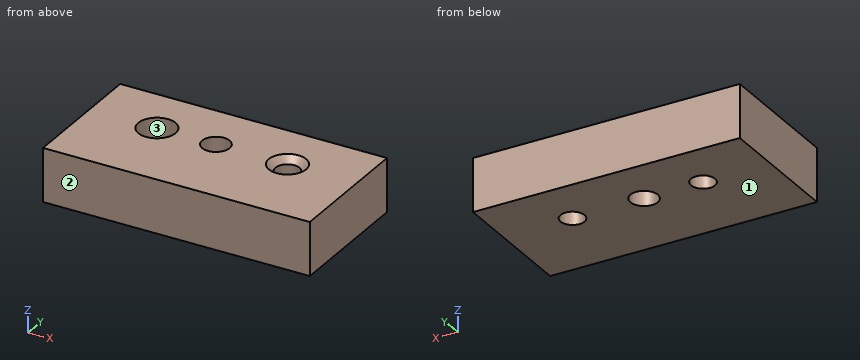
```python
from build123d import *

# Parameters (mm, degrees)
F0_W           = 100
F0_H           = 50
F1_DEPTH       = 20
F3_D           = 9
F3_DEPTH       = 30
F3_CBORE_D     = 14
F3_CBORE_DEPTH = 10
F3_TIP         = 2.7038727856
F4_D           = 9
F4_CSINK_D     = 14
F4_CSINK_ANGLE = 90
F5_D           = 10.3


with BuildPart() as f1:
    # F0 (on Top) → F1 (new body)
    with BuildSketch(Plane.XY):
        with Locations((19.3940885365, -5.1782257724)):
            Rectangle(F0_W, F0_H)
    extrude(amount=F1_DEPTH)

    # F3
    with Locations(Plane.XY.offset(20)):
        with Locations((-5.3611323237, 0)):
            CounterBoreHole(F3_D / 2, F3_CBORE_D / 2, F3_CBORE_DEPTH, depth=F3_DEPTH)
            with Locations((0, 0, -(F3_DEPTH + F3_TIP / 2))):  # 118° drill point
                Cone(0, F3_D / 2, F3_TIP, mode=Mode.SUBTRACT)

    # F4 (through all)
    with Locations(Plane.XY.offset(20)):
        with Locations((43.5566157103, 0)):
            CounterSinkHole(F4_D / 2, F4_CSINK_D / 2, counter_sink_angle=F4_CSINK_ANGLE)

    # F5 (through all)
    with Locations(Plane.XY.offset(20)):
        with Locations((16.7399458587, 0)):
            Hole(F5_D / 2)


solid = f1.part
```
Model file for the job. Use its own axes, mm. Face numbers are marked on the shaded views. Coordinates: 2 decimals unless noted, no trailing zeros. Order: outer loops, then holes, each group sorted by start corner. A loop starts at its lowest first (then second) coordinate and runs counter-clockwise, first axis right, second up. Notation, with made-up numbers: (55.5, 6.5) - (87.5, 6.5) arc R30 cw to (87.5, 34.5) - close; hole circle Ø7 at (55.25, -5). An arc over 180 degrees is marked (long way). Return JSON: item names as keys, results as strings. Group by question number.
1) Saw through at B-B, the plane z = 6.5. Write the cut outline in (x, y).
2) Saw through at A-A, the plane y = 0. Write the cut outline in (x, z), plus the area to 3 significant figures.
3) Saw through at C-C, the plane z = 15.25. Write the cut outline in (x, y), plus the area to 3 significant figures.
4) Flat gauge pins, fed straight in: P1, Ø8, axis at x = -5.36, y = 0, coming from the +Z side; P2, Ø7, axis at x = -6, y = 2, coming from the +Z side. Where does each tip first touch, or does it go through?
5) Mould opens along Y. For the marked faces 1, 2 and 3 say: released by +Y, released by -Y, zero draft, split by the parting line, or undercut.
6) Probe line 1 (X direction, y = -4, z = 17); line 2 (Y direction, x = 43, z = 5.25); line 3 (Y direction, x = 13.5, z = 14.5). List the from-to ranges inside material, lowest first. Write a range as from..to.
7) Saw through at D-D, the plane x = 0.5. Write the cut outline in (y, z).
Values found:
{
 "1": {"outline": "(-30.61, -30.18) - (69.39, -30.18) - (69.39, 19.82) - (-30.61, 19.82) - close; hole circle Ø9 at (-5.36, 0); hole circle Ø10.3 at (16.74, 0); hole circle Ø9 at (43.56, 0)"},
 "2": {"outline": "(-30.61, 0) - (-9.86, 0) - (-9.86, 10) - (-12.36, 10) - (-12.36, 20) - (-30.61, 20) - close; (-0.86, 0) - (11.59, 0) - (11.59, 20) - (1.64, 20) - (1.64, 10) - (-0.86, 10) - close; (21.89, 0) - (39.06, 0) - (39.06, 17.5) - (36.56, 20) - (21.89, 20) - close; (48.06, 0) - (69.39, 0) - (69.39, 20) - (50.56, 20) - (48.06, 17.5) - close", "area": "1,380 mm²"},
 "3": {"outline": "(-30.61, -30.18) - (69.39, -30.18) - (69.39, 19.82) - (-30.61, 19.82) - close; hole circle Ø14 at (-5.36, 0); hole circle Ø10.3 at (16.74, 0); hole circle Ø9 at (43.56, 0)", "area": "4,700 mm²"},
 "4": {"P1": "passes through", "P2": "stops at z = 10"},
 "5": {"face 1": "zero draft", "face 2": "released by -Y", "face 3": "undercut"},
 "6": {"line 1": "x = -30.61..-11.11, 0.38..13.5, 19.98..41.5, 45.62..69.39", "line 2": "y = -30.18..-4.47, 4.47..19.82", "line 3": "y = -30.18..-4, 4..19.82"},
 "7": {"outline": "(-30.18, 0) - (19.82, 0) - (19.82, 20) - (3.83, 20) - (3.83, 10) - (-3.83, 10) - (-3.83, 20) - (-30.18, 20) - close"}
}
